Input: part model. Units: mm. Frame: model coordinates. Face numbers are marked on the shaded views. Give positions to 0.01 mm unless a question says otherwise; leave off trailing zeros. Loops run counter-clockwise (first coordinate to the right, second up) from the corner with the lowest first, then second, coordinate; pieces in that order, holes last. Notation, with made-up numbers: M 88.5,-1 L 120.5,-1 A24 ccw 120.5,15 Z; hole C 22,66.25 d3. An arc over 180 degrees is marked long. Answer as a JSON object with one key per item and string values. Group by question number.
1) Draft query along X for the marked faces 1 and 2. Return one class per face: +X half, -X half, draft (parallel to the pull), parting line (faces both ways), or undercut.
2) Section query A-A on x = 9. Return loops of the section in (y, z).
3) Section query B-B on y = -1. Return loops of the section in (x, z), plus the area to 3 significant figures.
4) First-contact query: P1, Ø0.6, axis at x = 1, y = 1, coming from the +Z side; P2, Ø1.5, axis at y = 1.5, z = -7.5, coming from the -X side; P3, Ø2, axis at y = 0.5, z = -2, coming from the -X side. Flat tips, straight axial feed; report the tip coordinate or a pass-through.
5) Ray query, L1, parallel to Y at x = 15.5, z = 1; L2, parallel to X at y = -1.25, z = -5; L3, parallel to X at y = 0.75, z = -13.5. Return the intervals inside material, ascending.
from build123d import *

# Parameters (mm, degrees)
SKETCH1_R           = 1
BOSS_EXTRUDE1_DEPTH = 13
SKETCH2_R           = 1.75
SKETCH2_R_2         = 0.7
SKETCH2_R_3         = 0.75
BOSS_EXTRUDE2_DEPTH = 2
CIRPATTERN2_COUNT   = 3
SKETCH5_R           = 1.75
SKETCH5_R_2         = 0.5
BOSS_EXTRUDE3_DEPTH = 1
CUT_EXTRUDE1_REACH  = 33.393
CIRPATTERN3_COUNT   = 8


with BuildPart() as part:
    # Sketch1 → Boss-Extrude1 (new body)
    with BuildSketch(Plane(origin=(0, 0, 0), x_dir=(1, 0, 0), z_dir=(0, 1, 0))):
        with Locations(Location((0, -11, 0), (0, 0, 270))):
            Circle(SKETCH1_R)
    boss_extrude1 = extrude(amount=-BOSS_EXTRUDE1_DEPTH)

    # Sketch2 → Boss-Extrude2 (add)
    with BuildSketch(Plane(origin=(0, 0, 0), x_dir=(1, 0, 0), z_dir=(0, 1, 0))):
        with BuildLine():
            Line((-18, 1.5), (-15.929532322, 1.5))
            ThreePointArc((-15.929532322, 1.5), (-11.313708499, 11.313708499), (-1.5, 15.929532322))
            Line((-1.5, 15.929532322), (-1.5, 18))
            ThreePointArc((-1.5, 18), (0, 19.5), (1.5, 18))
            Line((1.5, 18), (1.5, 15.929532322))
            ThreePointArc((1.5, 15.929532322), (11.313708499, 11.313708499), (15.929532322, 1.5))
            Line((15.929532322, 1.5), (18, 1.5))
            ThreePointArc((18, 1.5), (19.5, 0), (18, -1.5))
            Line((18, -1.5), (15.929532322, -1.5))
            ThreePointArc((15.929532322, -1.5), (11.313708499, -11.313708499), (1.5, -15.929532322))
            Line((1.5, -15.929532322), (1.5, -18))
            ThreePointArc((1.5, -18), (0, -19.5), (-1.5, -18))
            Line((-1.5, -18), (-1.5, -15.929532322))
            ThreePointArc((-1.5, -15.929532322), (-11.313708499, -11.313708499), (-15.929532322, -1.5))
            Line((-15.929532322, -1.5), (-18, -1.5))
            ThreePointArc((-18, -1.5), (-19.5, 0), (-18, 1.5))
        make_face()
        with Locations(Location((0.8, 2.9, 0), (0, 0, 270))):
            Circle(SKETCH2_R, mode=Mode.SUBTRACT)
        with Locations(Location((0, 18, 0), (0, 0, 270))):
            Circle(SKETCH2_R_2, mode=Mode.SUBTRACT)
        with Locations(Location((18, 0, 0), (0, 0, 270))):
            Circle(SKETCH2_R_2, mode=Mode.SUBTRACT)
        with Locations(Location((-18, 0, 0), (0, 0, 270))):
            Circle(SKETCH2_R_2, mode=Mode.SUBTRACT)
        with Locations(Location((0, -18, 0), (0, 0, 270))):
            Circle(SKETCH2_R_2, mode=Mode.SUBTRACT)
        with Locations(Location((-5.7, -2, 0), (0, 0, 270))):
            Circle(SKETCH2_R_2, mode=Mode.SUBTRACT)
        with Locations(Location((5.7, -2, 0), (0, 0, 270))):
            Circle(SKETCH2_R_3, mode=Mode.SUBTRACT)
        with BuildLine():
            Line((-5.2, 3), (-5.2, 1))
            ThreePointArc((-5.2, 1), (-5.346446609, 0.646446609), (-5.7, 0.5))
            ThreePointArc((-5.7, 0.5), (-8.2, -2), (-5.7, -4.5))
            ThreePointArc((-5.7, -4.5), (-5.346446609, -4.646446609), (-5.2, -5))
            Line((-5.2, -5), (-5.2, -7))
            ThreePointArc((-5.2, -7), (-5.346446609, -7.353553391), (-5.7, -7.5))
            ThreePointArc((-5.7, -7.5), (-11.2, -2), (-5.7, 3.5))
            ThreePointArc((-5.7, 3.5), (-5.346446609, 3.353553391), (-5.2, 3))
        make_face(mode=Mode.SUBTRACT)
        with BuildLine():
            Line((2.934458944, -1.292677422), (2.934458944, -8.449761431))
            ThreePointArc((2.934458944, -8.449761431), (2.788012334, -8.803314822), (2.434458944, -8.949761431))
            Line((2.434458944, -8.949761431), (-2.434458944, -8.949761431))
            ThreePointArc((-2.434458944, -8.949761431), (-2.788012334, -8.803314822), (-2.934458944, -8.449761431))
            Line((-2.934458944, -8.449761431), (-2.934458944, -0.228621956))
            ThreePointArc((-2.934458944, -0.228621956), (-2.621952726, 0.234892965), (-2.075074617, 0.119002706))
            ThreePointArc((-2.075074617, 0.119002706), (-0.054005989, -1.007770947), (2.252852394, -0.826824375))
            ThreePointArc((2.252852394, -0.826824375), (2.716590762, -0.87988009), (2.934458944, -1.292677422))
        make_face(mode=Mode.SUBTRACT)
        with BuildLine():
            Line((-2.434458944, 8.949761431), (2.434458944, 8.949761431))
            ThreePointArc((2.434458944, 8.949761431), (2.788012334, 8.803314822), (2.934458944, 8.449761431))
            Line((2.934458944, 8.449761431), (2.934458944, 7.092677422))
            ThreePointArc((2.934458944, 7.092677422), (2.716590762, 6.67988009), (2.252852394, 6.626824375))
            ThreePointArc((2.252852394, 6.626824375), (-0.054005989, 6.807770947), (-2.075074617, 5.680997294))
            ThreePointArc((-2.075074617, 5.680997294), (-2.621952726, 5.565107035), (-2.934458944, 6.028621956))
            Line((-2.934458944, 6.028621956), (-2.934458944, 8.449761431))
            ThreePointArc((-2.934458944, 8.449761431), (-2.788012334, 8.803314822), (-2.434458944, 8.949761431))
        make_face(mode=Mode.SUBTRACT)
        with BuildLine():
            Line((5.2, -5), (5.2, -7))
            ThreePointArc((5.2, -7), (5.346446609, -7.353553391), (5.7, -7.5))
            ThreePointArc((5.7, -7.5), (11.2, -2), (5.7, 3.5))
            ThreePointArc((5.7, 3.5), (5.346446609, 3.353553391), (5.2, 3))
            Line((5.2, 3), (5.2, 1))
            ThreePointArc((5.2, 1), (5.346446609, 0.646446609), (5.7, 0.5))
            ThreePointArc((5.7, 0.5), (8.2, -2), (5.7, -4.5))
            ThreePointArc((5.7, -4.5), (5.346446609, -4.646446609), (5.2, -5))
        make_face(mode=Mode.SUBTRACT)
    extrude(amount=BOSS_EXTRUDE2_DEPTH)

    # CirPattern2: Boss-Extrude1 ×3 about axis
    cirpattern2_axis = Axis((0, 0, 0), (0, 1, 0))
    for i in range(1, CIRPATTERN2_COUNT):
        add(boss_extrude1.rotate(cirpattern2_axis, i * 360 / CIRPATTERN2_COUNT))

    # Sketch5 → Boss-Extrude3 (add)
    with BuildSketch(Plane.XZ):
        with Locations(Location((0.8, -2.9, 0), (0, 0, 270))):
            Circle(SKETCH5_R)
        with Locations(Location((0.8, -2.9, 0), (0, 0, 270))):
            Circle(SKETCH5_R_2, mode=Mode.SUBTRACT)
    extrude(amount=-BOSS_EXTRUDE3_DEPTH)

    # Sketch8 → Cut-Extrude1 (cut, up to next)
    with BuildSketch(Plane(origin=(0, 2, 0), x_dir=(1, 0, 0), z_dir=(0, 1, 0)), mode=Mode.PRIVATE) as cut_extrude1_sk1:
        with BuildLine():
            Line((4.176910704, 12.28097457), (4.551006159, 13.213456818))
            ThreePointArc((4.551006159, 13.213456818), (4.537914561, 13.615582258), (4.232825837, 13.877874327))
            ThreePointArc((4.232825837, 13.877874327), (0, 14.509038921), (-4.232825837, 13.877874327))
            ThreePointArc((-4.232825837, 13.877874327), (-4.537914561, 13.615582258), (-4.551006159, 13.213456818))
            Line((-4.551006159, 13.213456818), (-4.176910704, 12.28097457))
            ThreePointArc((-4.176910704, 12.28097457), (-3.930304731, 12.016900024), (-3.570150171, 11.987942034))
            ThreePointArc((-3.570150171, 11.987942034), (0, 12.508266325), (3.570150171, 11.987942034))
            ThreePointArc((3.570150171, 11.987942034), (3.930304731, 12.016900024), (4.176910704, 12.28097457))
        make_face()
    cut_extrude1_tool1 = extrude(cut_extrude1_sk1.sketch, amount=-CUT_EXTRUDE1_REACH, mode=Mode.PRIVATE) & part.part
    cut_extrude1 = cut_extrude1_tool1.solids().sort_by_distance((0, 2, -13.296858))[0]
    add(cut_extrude1, mode=Mode.SUBTRACT)

    # CirPattern3: Cut-Extrude1 ×8 about axis
    cirpattern3_axis = Axis((0, 0, 0), (0, 1, 0))
    for i in range(1, CIRPATTERN3_COUNT):
        add(cut_extrude1.rotate(cirpattern3_axis, i * 360 / CIRPATTERN3_COUNT), mode=Mode.SUBTRACT)


solid = part.part
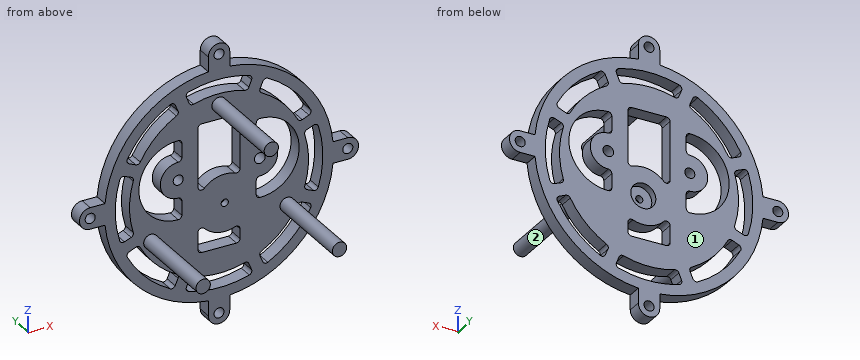
Output:
{
 "1": {"face 1": "draft", "face 2": "undercut"},
 "2": {"outline": "M -13,-6.35 L 0,-6.35 L 0,-8.69 L 2,-8.69 L 2,-2.4 L 0,-2.4 L 0,-4.65 L -13,-4.65 Z; M 0,-13.23 L 2,-13.23 L 2,-11.38 L 0,-11.38 Z; M 0,6.4 L 2,6.4 L 2,8.69 L 0,8.69 Z; M 0,11.38 L 2,11.38 L 2,13.23 L 0,13.23 Z"},
 "3": {"outline": "C -9.53,-5.5 d2; C 0,11 d2; C 9.53,-5.5 d2", "area": "9.42 mm^2"},
 "4": {"P1": "stops at z = 19.33", "P2": "stops at x = -14.51", "P3": "stops at x = -19.12"},
 "5": {"L1": "y = 0 to 2", "L2": "x = -10.39 to -8.66, 8.66 to 10.39", "L3": "x = -8.59 to -4.58, 4.58 to 8.59"}
}
